The model under review builds one solid part; all positions refer to its coordinate system, in mm. A direction names the side the tool comes from. Round coordinates to 2 decimals unless told otherwise and drop trailing zeros. Loops run counter-clockwise (first coordinate to the right, second up) from the corner with the lowest first, then second, coordinate; pieces in that order, holes last. Notation, with made-up numbers: M 48,-25 L 76,-25 A16 ccw 76,4 Z; hole C 72,-27 d2. An arc over 180 degrees is marked long. Return JSON: item names as keys, results as strings. Group by question number.
Q1. Consider section A-A (x = 88). State the section outline as (y, z) points, and give its area (3 significant figures).
Q2. Consider section B-B (z = 60.25). State the section outline as (x, y) points.
Q3. Consider section C-C (y = -43). State the section outline as (x, z) points, and give its area (3 significant figures).
Q4. Clearance check with flat-ended pins moving along their axes: pin 1 Ø1.8 at (x, y) = (69.5, -34.5) entering from -Z; pin 2 Ø5 at (x, z) = (59, 57.5) entering from +Y; pin 3 Ø5 at (x, y) = (81, -38) entering from -Z; pin 4 Ø5 at (y, z) = (-56.5, 60.5) entering from +X. State where each tip first meets the part, or that it passes through.
Q5. To check wall thickness, follow line 1 along Y through (x, z) = (85, 64.5); line 2 along Y through (x, z) = (78.5, 64); line 3 along X through (y, z) = (-80, 62.75). State the ranges of each line that lie inside material, in increasing order.
Q6. Draft analysis for pull direction Y (two halves, no side actions). For faces 1 (the face through (75.638, -101.094, 56.479)), 2 (the face through (87.35, -50.59, 55.99)), 3 (the face through (59, -90, 55)), state which applies: pulls with the +Y half, pulls with the -Y half, needs draft (parallel to the pull), parting line crosses it, or undercut.
Q7. Consider section D-D (x = 41). State the section outline as (y, z) points, and give its area (3 significant figures).
Q8. For faces 4 (the face through (53.122, -82.819, 59.93)), 5 (the face through (65.72, -35.53, 56.48)), 6 (the face through (90.31, -90.01, 55.51)), list the 3-axis set-ups (+Z, -Z, +X, -X, +Y, -Y) from which the entire face can be reached by the end or side of a thin tool; tool diameter is ignored.
from build123d import *

# Parameters (mm, degrees)
CYLINDER1730_R              = 3
CYLINDER1730_DEPTH          = 3
CYLINDER1727_R              = 3
CYLINDER1727_DEPTH          = 3
CYLINDER1728_R              = 3
CYLINDER1728_DEPTH          = 3
CYLINDER1729_R              = 3
CYLINDER1729_DEPTH          = 3
COMPOUND871_PLACEMENT_ANGLE = 225
CYLINDER1734_R              = 1.5
CYLINDER1734_DEPTH          = 60
CYLINDER1731_R              = 1.5
CYLINDER1731_DEPTH          = 60
CYLINDER1732_R              = 1.5
CYLINDER1732_DEPTH          = 60
CYLINDER1733_R              = 1.5
CYLINDER1733_DEPTH          = 60
COMPOUND874_PLACEMENT_ANGLE = 225
CYLINDER1735_R              = 74
CYLINDER1735_DEPTH          = 40
BOX688_W                    = 42
BOX688_H                    = 62
BOX688_DEPTH                = 50
COMPOUND872_PLACEMENT_ANGLE = 225
BOX689_W                    = 54
BOX689_H                    = 68
BOX689_DEPTH                = 10
COMPOUND873_PLACEMENT_ANGLE = 225
CHAMFER054_SIZE             = 3
CHAMFER055_SIZE             = 2
CHAMFER056_SIZE             = 1


with BuildPart() as obj1:
    # Cylinder1730 → Cylinder1730 (new body)
    with BuildSketch(Plane(origin=(-24, 73, -80), x_dir=(1, 0, 0), z_dir=(0, 0, 1))):
        Circle(CYLINDER1730_R)
    extrude(amount=CYLINDER1730_DEPTH)


with BuildPart() as obj2:
    # Cylinder1727 → Cylinder1727 (new body)
    with BuildSketch(Plane(origin=(-15, 125, -80), x_dir=(1, 0, 0), z_dir=(0, 0, 1))):
        Circle(CYLINDER1727_R)
    extrude(amount=CYLINDER1727_DEPTH)


with BuildPart() as obj3:
    # Cylinder1728 → Cylinder1728 (new body)
    with BuildSketch(Plane(origin=(15, 125, -80), x_dir=(1, 0, 0), z_dir=(0, 0, 1))):
        Circle(CYLINDER1728_R)
    extrude(amount=CYLINDER1728_DEPTH)


with BuildPart() as compound871:
    # Cylinder1729 → Cylinder1729 (new body)
    with BuildSketch(Plane(origin=(24, 73, -80), x_dir=(1, 0, 0), z_dir=(0, 0, 1))):
        Circle(CYLINDER1729_R)
    extrude(amount=CYLINDER1729_DEPTH)

    # Compound871: union obj1, obj2, obj3
    add(obj1.part)
    add(obj2.part)
    add(obj3.part)


with BuildPart() as compound871_1:
    # Compound871 placement: moved
    add(compound871.part.moved(Location((0, 0, 135))).rotate(Axis((0, 0, 135), (0, 0, 1)), COMPOUND871_PLACEMENT_ANGLE))


with BuildPart() as obj4:
    # Cylinder1734 → Cylinder1734 (new body)
    with BuildSketch(Plane(origin=(-24, 73, -80), x_dir=(1, 0, 0), z_dir=(0, 0, 1))):
        Circle(CYLINDER1734_R)
    extrude(amount=CYLINDER1734_DEPTH)


with BuildPart() as obj5:
    # Cylinder1731 → Cylinder1731 (new body)
    with BuildSketch(Plane(origin=(-15, 125, -80), x_dir=(1, 0, 0), z_dir=(0, 0, 1))):
        Circle(CYLINDER1731_R)
    extrude(amount=CYLINDER1731_DEPTH)


with BuildPart() as obj6:
    # Cylinder1732 → Cylinder1732 (new body)
    with BuildSketch(Plane(origin=(15, 125, -80), x_dir=(1, 0, 0), z_dir=(0, 0, 1))):
        Circle(CYLINDER1732_R)
    extrude(amount=CYLINDER1732_DEPTH)


with BuildPart() as compound874:
    # Cylinder1733 → Cylinder1733 (new body)
    with BuildSketch(Plane(origin=(24, 73, -80), x_dir=(1, 0, 0), z_dir=(0, 0, 1))):
        Circle(CYLINDER1733_R)
    extrude(amount=CYLINDER1733_DEPTH)

    # Compound874: union obj4, obj5, obj6
    add(obj4.part)
    add(obj5.part)
    add(obj6.part)


with BuildPart() as compound874_1:
    # Compound874 placement: moved
    add(compound874.part.moved(Location((0, 0, 100))).rotate(Axis((0, 0, 100), (0, 0, 1)), COMPOUND874_PLACEMENT_ANGLE))


with BuildPart() as obj7:
    # Cylinder1735 → Cylinder1735 (new body)
    with BuildSketch(Plane.XY.offset(44)):
        Circle(CYLINDER1735_R)
    extrude(amount=CYLINDER1735_DEPTH)


with BuildPart() as compound872:
    # Box688 → Box688 (new body)
    with BuildSketch(Plane(origin=(-21.001071, 60.005081, 31), x_dir=(1, 0, 0), z_dir=(0, 0, 1))):
        with Locations((21, 31)):
            Rectangle(BOX688_W, BOX688_H)
    extrude(amount=BOX688_DEPTH)


with BuildPart() as compound872_1:
    # Compound872 placement: moved
    add(compound872.part.rotate(Axis((0, 0, 0), (0, 0, 1)), COMPOUND872_PLACEMENT_ANGLE))


with BuildPart() as cut512:
    # Box689 → Box689 (new body)
    with BuildSketch(Plane(origin=(-27.004408, 59.99801, 75), x_dir=(1, 0, 0), z_dir=(0, 0, 1))):
        with Locations((27, 34)):
            Rectangle(BOX689_W, BOX689_H)
    extrude(amount=BOX689_DEPTH)


with BuildPart() as cut512_1:
    # Compound873 placement: moved
    add(cut512.part.moved(Location((0, 0, -20))).rotate(Axis((0, 0, -20), (0, 0, 1)), COMPOUND873_PLACEMENT_ANGLE))

    # Cut502: cut Compound872
    add(compound872_1.part, mode=Mode.SUBTRACT)

    # Cut510: cut obj7
    add(obj7.part, mode=Mode.SUBTRACT)

    # Chamfer054
    chamfer054_edges = [cut512_1.edges().sort_by_distance(p)[0] for p in [
        (109.603261, -71.413261, 60),
        (71.419495, -109.597027, 60),
    ]]
    chamfer(chamfer054_edges, length=CHAMFER054_SIZE)

    # Chamfer055
    chamfer055_edges = [cut512_1.edges().sort_by_distance(p)[0] for p in [
        (87.647149, -49.457149, 55),
        (49.464605, -87.642137, 55),
    ]]
    chamfer(chamfer055_edges, length=CHAMFER055_SIZE)

    # Chamfer056
    chamfer056_edges = [cut512_1.edges().sort_by_distance(p)[0] for p in [
        (90.511378, -90.505144, 55),
    ]]
    chamfer(chamfer056_edges, length=CHAMFER056_SIZE)

    # Cut511: cut Compound874
    add(compound874_1.part, mode=Mode.SUBTRACT)

    # Cut512: cut Compound871
    add(compound871_1.part, mode=Mode.SUBTRACT)


solid = cut512_1.part
Values:
{
 "1": {"outline": "M -93.02,56 L -91.6,55 L -84.54,55 L -84.54,65 L -93.02,65 Z; M -58.3,55 L -52.64,55 L -49.81,57 L -49.81,65 L -58.3,65 Z", "area": "166 mm2"},
 "2": {"outline": "M 29.63,-67.81 L 69.3,-107.48 L 73.54,-107.48 L 107.48,-73.53 L 107.48,-69.29 L 67.81,-29.62 A74 cw 65.02,-35.32 L 101.12,-71.42 L 71.42,-101.12 L 35.33,-65.02 A74 cw Z; hole C 34.65,-68.59 d3; hole C 68.59,-34.65 d3; hole C 77.78,-98.99 d3; hole C 98.99,-77.78 d3"},
 "3": {"outline": "M 72.7,55 L 78.36,55 L 81.19,57 L 81.19,65 L 72.7,65 Z", "area": "82.1 mm2"},
 "4": {"pin 1": "stops at z = 58", "pin 2": "stops at y = -86.2", "pin 3": "passes through", "pin 4": "stops at x = 97.19"},
 "5": {"line 1": "y = -96.02 to -87.54, -55.3 to -46.81", "line 2": "y = -102.52 to -100.31, -97.68 to -94.04, -48.8 to -40.31", "line 3": "x = 41.82 to 50.3, 92.54 to 101.02"},
 "6": {"face 1": "undercut", "face 2": "pulls with the +Y half", "face 3": "needs draft"},
 "7": {"outline": "M -79.18,57 L -76.35,55 L -70.7,55 L -70.7,65 L -79.18,65 Z", "area": "82.0 mm2"},
 "8": {"face 4": "+Z, -Z", "face 5": "-Z", "face 6": "-Z, +X, -Y"}
}
